from build123d import *

# Parameters (mm, degrees)
SKETCH4_R          = 4.15
CUT_EXTRUDE1_DEPTH = 15
CHAMFER1_SIZE      = 1.5
CUT_EXTRUDE2_DEPTH = 1.5875


with BuildPart() as part:
    # Sketch1 → Revolve1 (revolve)
    with BuildSketch(Plane.XY):
        Polygon((-67, 0), (67, 0), (67, 11), (42, 11), (42, 9.5), (-28, 9.5), (-28, 7.9375), (-67, 7.9375), align=None)
    revolve(axis=Axis((-84.93546187, 0, 0), (1, 0, 0)))

    # Sketch2 → 1/8 NPT Tapped Hole1 (revolve, cut)
    with BuildSketch(Plane(origin=(67, 0, 0), x_dir=(0, 0, -1), z_dir=(0, 1, 0))):
        Polygon((0, 0), (0, 46.533468714), (4.2164, 44), (4.2164, 6.92404), (4.53740497, 6.92404), (4.74472, 0), align=None)
    revolve(axis=Axis((73.35, 0, 0), (-1, 0, 0)), mode=Mode.SUBTRACT)

    # Sketch4 → Cut-Extrude1 (cut, symmetric)
    with BuildSketch(Plane(origin=(0, 0, 0), x_dir=(1, 0, 0), z_dir=(0, 1, 0))):
        with Locations((28, 0)):
            Circle(SKETCH4_R)
    extrude(amount=CUT_EXTRUDE1_DEPTH, both=True, mode=Mode.SUBTRACT)

    # Chamfer1
    chamfer1_edges = [part.edges().sort_by_distance(p)[0] for p in [
        (-67, -7.9375, 0),
    ]]
    chamfer(chamfer1_edges, length=CHAMFER1_SIZE)

    # Sketch7 → Cut-Extrude2 (cut, symmetric)
    with BuildSketch(Plane.XY):
        with BuildLine():
            Line((-48.391776656, 9.525), (-29.608223344, 9.525))
            ThreePointArc((-29.608223344, 9.525), (-39, 1.5875), (-48.391776656, 9.525))
        make_face()
    extrude(amount=CUT_EXTRUDE2_DEPTH, both=True, mode=Mode.SUBTRACT)


solid = part.part
CAD build for the part. Positions are in the model's coordinates, mm. A direction names the side the tool comes from. Give positions to 0.01 mm unless a question says otherwise; leave off trailing zeros. Loops run counter-clockwise (first coordinate to the right, second up) from the corner with the lowest first, then second, coordinate; pieces in that order, holes last. Notation, with made-up numbers: M 7.5,71 L 11.5,71 A4 cw 11.5,77 Z; hole C -9,45.25 d2. An arc over 180 degrees is marked long. Answer in a Markdown table with one row per item. Add a question column.
Item 1: Band-saw the part on A-A on x = 28.5. Give the cut face in (y, z), then the cut area to 3 significant figures.
Item 2: Tool access for faces 4 (the face through (-39, 5, 1.588)), 5 (the face through (-28, -2, -8)), 6 (the face through (45.9, 1.6, -3.9)): list every direction of +Z, -Z, +X, -X, +Y, -Y with a clear straight run to the whole face (end or side of a thin tool).
Item 3: Mould opens along X. For faces 1 (the face through (63.59, 4.53, 1.01)), 2 (the face through (-38.84, 1.59, 0.02)), 3 (the face through (-67, 0, 0)) say: +X half, -X half, draft (parallel to the pull), parting line (faces both ways), or undercut.
Item 4: Probe probe 1 along Z at (x, y) = (51, 0); probe 2 along Z at (x, y) = (39, 0); probe 3 along X at (y, z) = (7, 0). List the from-to ranges inside material, lowest first.
Item 5: Band-saw the part on B-B on x = -37. Give the cut face in (y, z) (1 decimal), then the cut area to 3 significant figures.
Item 6: Drop flat-ended pins along their axis: P1, Ø8, axis at x = -2.5, y = 1.5, coming from the +Z side; P2, Ø7, axis at x = -35, y = 5, coming from the +Z side; P3, Ø5, axis at x = -11.5, z = -1, coming from the -Y side; P4, Ø10, axis at y = -1.5, z = 1, coming from the +X side. Give the stop position or say it passes through.
Reply:
| question | item | result |
|---|---|---|
| 1 | outline | M -8.56,-4.12 A9.5 ccw 8.56,-4.12 L 0.9,-4.12 A4.22 cw -0.9,-4.12 Z; M -8.56,4.12 L -0.9,4.12 A4.22 cw 0.9,4.12 L 8.56,4.12 A9.5 ccw Z |
| 1 | area | 132 mm^2 |
| 2 | face 4 | +Y |
| 2 | face 5 | -X |
| 2 | face 6 | +X |
| 3 | face 1 | +X half |
| 3 | face 2 | undercut |
| 3 | face 3 | -X half |
| 4 | probe 1 | z = -11 to -4.22, 4.22 to 11 |
| 4 | probe 2 | z = -9.5 to -4.22, 4.22 to 9.5 |
| 4 | probe 3 | x = -66.44 to -47.59, -30.41 to 23.85, 32.15 to 67 |
| 5 | outline | M 1.8,-1.6 L 1.8,1.6 L 7.8,1.6 A7.9 ccw long 7.8,-1.6 Z |
| 5 | area | 179 mm^2 |
| 6 | P1 | stops at z = 9.5 |
| 6 | P2 | stops at z = 7.79 |
| 6 | P3 | stops at y = -9.5 |
| 6 | P4 | stops at x = 67 |
